Source: CAD feature listing. Evaluate the final solid. Frame: model axes, mm. Give positions to 0.01 mm unless a question says otherwise; leave off trailing zeros. Write each loop counter-clockwise with the first axis right and the second up, starting at its lowest first coordinate (ties: lowest second). Pieces come first, ordered by that corner, then holes. Notation, with made-up numbers: M 73.25,63.5 L 114.25,63.5 A8 cw 114.25,67.5 Z; hole C -15,40 d3. An arc over 180 degrees is marked long. Return JSON: item names as keys, results as strings.
```python
from build123d import *

# Parameters (mm, degrees)
PAD_DEPTH    = 3
PAD001_DEPTH = 1


with BuildPart() as part:
    # Sketch → Pad (new body)
    with BuildSketch(Plane.XY):
        Polygon((-143.5, 11.5), (-143.5, -11.5), (-16, -11.5), (-16, -9.5), (16, -9.5), (16, -11.5), (143.5, -11.5), (143.5, 11.5), align=None)
    extrude(amount=PAD_DEPTH)

    # Sketch001 (on Face9 of Pad) → Pad001 (join)
    with BuildSketch(Plane(origin=(0, 0, 0), x_dir=(1, 0, 0), z_dir=(0, 0, -1))):
        Polygon((-143.5, 11.5), (-143.5, -13.5), (143.5, -13.5), (143.5, 11.5), (16, 11.5), (16, 9.5), (-16, 9.5), (-16, 11.5), align=None)
    extrude(amount=-PAD001_DEPTH)


solid = part.part
```
1) Cut plane C-C, the plane x = 11.5. Return the cut outline in (y, z), then the cut area to 3 significant figures.
Numbers:
{"outline": "M -9.5,0 L 13.5,0 L 13.5,1 L 11.5,1 L 11.5,3 L -9.5,3 Z", "area": "65.0 mm²"}
2) Contact query for flat-ended pins moving along their axis: pin 1 Ø1.6 at (x, z) = (-62, 2.5) entering from +Y; pin 2 Ø1 at (x, y) = (-29, 13) entering from +Z; pin 3 Ø0.9 at (x, z) = (2, 1.5) entering from -Y. Output: stop coordinate, or through.
Numbers:
{"pin 1": "stops at y = 11.5", "pin 2": "stops at z = 1", "pin 3": "stops at y = -9.5"}
3) Cut plane A-A, the plane z = 1.9. Return the cut outline in (x, y).
Numbers:
{"outline": "M -143.5,-11.5 L -16,-11.5 L -16,-9.5 L 16,-9.5 L 16,-11.5 L 143.5,-11.5 L 143.5,11.5 L -143.5,11.5 Z"}
4) Line query: line 1 (Y direction, x = -61, z = 2.35); line 2 (Y direction, x = 1, z = 2.2). Output: solid intervals per line, ascending. Write a range as [from, to].
Numbers:
{"line 1": "y = [-11.5, 11.5]", "line 2": "y = [-9.5, 11.5]"}
5) Cut plane B-B, the plane x = -51.5. Return the cut outline in (y, z).
Numbers:
{"outline": "M -11.5,0 L 13.5,0 L 13.5,1 L 11.5,1 L 11.5,3 L -11.5,3 Z"}
